The model under review builds one solid part; all positions refer to its coordinate system, in mm. Give positions to 0.01 mm unless a question says otherwise; leave off trailing zeros. Loops run counter-clockwise (first coordinate to the right, second up) from the corner with the lowest first, then second, coordinate; pieces in that order, holes last. Notation, with made-up numbers: (70.5, -19) - (110.5, -19) arc R20 ccw to (110.5, -9) - close; hole circle Ø4 at (44, 28). An arc over 180 degrees is marked (long way). Answer as a JSON object with one key per item and string values.
from build123d import *

# Parameters (mm, degrees)
F1_DEPTH = 1


# Not quite as in the source:
# - ends of sketch curves that miss each other by under 0.0002 mm in the source are joined


with BuildPart() as f1:
    # F0 (on Top) → F1 (new body)
    with BuildSketch(Plane.XY):
        with BuildLine():
            ThreePointArc((5.1893277963, 10.709786768), (5.015248305, 11.2735733528), (4.5536171698, 11.6410725739))
            ThreePointArc((4.5536171698, 11.6410725739), (0, 12.5), (-4.5536171698, 11.6410725739))
            ThreePointArc((-4.5536171698, 11.6410725739), (-5.015248305, 11.2735733528), (-5.1893277963, 10.709786768))
            Line((-5.1893277963, 10.709786768), (-5.1893277963, 10.5791593824))
            ThreePointArc((-5.1893277963, 10.5791593824), (-5.3218672589, 10.0816533863), (-5.6843522286, 9.716025745))
            ThreePointArc((-5.6843522286, 9.716025745), (-7.9596801612, 7.9596801612), (-9.716025745, 5.6843522286))
            ThreePointArc((-9.716025745, 5.6843522286), (-10.0816533863, 5.3218672589), (-10.5791593824, 5.1893277963))
            Line((-10.5791593824, 5.1893277963), (-10.709786768, 5.1893277963))
            ThreePointArc((-10.709786768, 5.1893277963), (-11.2735733528, 5.015248305), (-11.6410725739, 4.5536171698))
            ThreePointArc((-11.6410725739, 4.5536171698), (-12.5, 0), (-11.6410725739, -4.5536171698))
            ThreePointArc((-11.6410725739, -4.5536171698), (-11.2735733528, -5.015248305), (-10.709786768, -5.1893277963))
            Line((-10.709786768, -5.1893277963), (-10.5791593824, -5.1893277963))
            ThreePointArc((-10.5791593824, -5.1893277963), (-10.0816533863, -5.3218672589), (-9.716025745, -5.6843522286))
            ThreePointArc((-9.716025745, -5.6843522286), (-7.9596801612, -7.9596801612), (-5.6843522286, -9.716025745))
            ThreePointArc((-5.6843522286, -9.716025745), (-5.3218672589, -10.0816533863), (-5.1893277963, -10.5791593824))
            Line((-5.1893277963, -10.5791593824), (-5.1893277963, -10.709786768))
            ThreePointArc((-5.1893277963, -10.709786768), (-5.015248305, -11.2735733528), (-4.5536171698, -11.6410725739))
            ThreePointArc((-4.5536171698, -11.6410725739), (0, -12.5), (4.5536171698, -11.6410725739))
            ThreePointArc((4.5536171698, -11.6410725739), (5.015248305, -11.2735733528), (5.1893277963, -10.709786768))
            Line((5.1893277963, -10.709786768), (5.1893277963, -10.5791593824))
            ThreePointArc((5.1893277963, -10.5791593824), (5.3218672589, -10.0816533863), (5.6843522286, -9.716025745))
            ThreePointArc((5.6843522286, -9.716025745), (7.9596801612, -7.9596801612), (9.716025745, -5.6843522286))
            ThreePointArc((9.716025745, -5.6843522286), (10.0816533863, -5.3218672589), (10.5791593824, -5.1893277963))
            Line((10.5791593824, -5.1893277963), (10.709786768, -5.1893277963))
            ThreePointArc((10.709786768, -5.1893277963), (11.2735733528, -5.015248305), (11.6410725739, -4.5536171698))
            ThreePointArc((11.6410725739, -4.5536171698), (12.5, 0), (11.6410725739, 4.5536171698))
            ThreePointArc((11.6410725739, 4.5536171698), (11.2735733528, 5.015248305), (10.709786768, 5.1893277963))
            Line((10.709786768, 5.1893277963), (10.5791593824, 5.1893277963))
            ThreePointArc((10.5791593824, 5.1893277963), (10.0816533863, 5.3218672589), (9.716025745, 5.6843522286))
            ThreePointArc((9.716025745, 5.6843522286), (7.9596801612, 7.9596801612), (5.6843522286, 9.716025745))
            ThreePointArc((5.6843522286, 9.716025745), (5.3218672589, 10.0816533863), (5.1893277963, 10.5791593824))
            Line((5.1893277963, 10.5791593824), (5.1893277963, 10.709786768))
        make_face()
        with BuildLine():
            Line((-1.7389636828, -9.696227699), (-1.7389636828, -7.803772301))
            ThreePointArc((-1.7389636828, -7.803772301), (0, -6.0648086182), (1.7389636828, -7.803772301))
            Line((1.7389636828, -7.803772301), (1.7389636828, -9.696227699))
            ThreePointArc((1.7389636828, -9.696227699), (0, -11.4351913818), (-1.7389636828, -9.696227699))
        make_face(mode=Mode.SUBTRACT)
        with BuildLine():
            Line((-4.0980324058, 1.6278386791), (-4.596886989, 2.1259958547))
            Line((-4.596886989, 2.1259958547), (-7.2887076389, 4.8140532918))
            ThreePointArc((-7.2887076389, 4.8140532918), (-7.2895746597, 7.2895734489), (-4.8140532909, 7.2887076381))
            Line((-4.8140532909, 7.2887076381), (-2.1259958547, 4.596886989))
            Line((-2.1259958547, 4.596886989), (-1.6278386791, 4.0980324058))
            ThreePointArc((-1.6278386791, 4.0980324058), (-1.5783462567, 4.0709813489), (-1.5220880269, 4.0750150967))
            ThreePointArc((-1.5220880269, 4.0750150967), (0.0320676528, 4.349881799), (1.5820019575, 4.052131514))
            Line((1.5820019575, 4.052131514), (2.1259958547, 4.596886989))
            Line((2.1259958547, 4.596886989), (4.8140532909, 7.2887076381))
            ThreePointArc((4.8140532909, 7.2887076381), (7.2895746597, 7.2895734489), (7.2887088489, 4.8140520801))
            Line((7.2887088489, 4.8140520801), (4.596886989, 2.1259958547))
            Line((4.596886989, 2.1259958547), (4.0980324058, 1.6278386791))
            ThreePointArc((4.0980324058, 1.6278386791), (4.0709813489, 1.5783462567), (4.0750150967, 1.5220880269))
            ThreePointArc((4.0750150967, 1.5220880269), (4.35, 0), (4.0750150967, -1.5220880269))
            ThreePointArc((4.0750150967, -1.5220880269), (4.0709813489, -1.5783462567), (4.0980324058, -1.6278386791))
            Line((4.0980324058, -1.6278386791), (4.596886989, -2.1259958547))
            Line((4.596886989, -2.1259958547), (7.2887076389, -4.8140532918))
            ThreePointArc((7.2887076389, -4.8140532918), (7.2904398646, -7.2887076385), (4.8157843062, -7.2904386534))
            Line((4.8157843062, -7.2904386534), (4.8140532909, -7.2887076381))
            Line((4.8140532909, -7.2887076381), (2.1259958547, -4.596886989))
            Line((2.1259958547, -4.596886989), (1.6278386791, -4.0980324058))
            ThreePointArc((1.6278386791, -4.0980324058), (1.5783462567, -4.0709813489), (1.5220880269, -4.0750150967))
            ThreePointArc((1.5220880269, -4.0750150967), (0, -4.35), (-1.5220880269, -4.0750150967))
            ThreePointArc((-1.5220880269, -4.0750150967), (-1.5783462567, -4.0709813489), (-1.6278386791, -4.0980324058))
            Line((-1.6278386791, -4.0980324058), (-2.1259958547, -4.596886989))
            Line((-2.1259958547, -4.596886989), (-4.8140532909, -7.2887076381))
            ThreePointArc((-4.8140532909, -7.2887076381), (-7.2895746597, -7.2895734489), (-7.2887088489, -4.8140520801))
            Line((-7.2887088489, -4.8140520801), (-4.596886989, -2.1259958547))
            Line((-4.596886989, -2.1259958547), (-4.0980324058, -1.6278386791))
            ThreePointArc((-4.0980324058, -1.6278386791), (-4.0709813489, -1.5783462567), (-4.0750150967, -1.5220880269))
            ThreePointArc((-4.0750150967, -1.5220880269), (-4.35, 0), (-4.0750150967, 1.5220880269))
            ThreePointArc((-4.0750150967, 1.5220880269), (-4.0709813489, 1.5783462567), (-4.0980324058, 1.6278386791))
        make_face(mode=Mode.SUBTRACT)
        with BuildLine():
            Line((-7.803772301, -1.7389636828), (-9.696227699, -1.7389636828))
            ThreePointArc((-9.696227699, -1.7389636828), (-11.4351913818, 0), (-9.696227699, 1.7389636828))
            Line((-9.696227699, 1.7389636828), (-7.803772301, 1.7389636828))
            ThreePointArc((-7.803772301, 1.7389636828), (-6.0648086182, 0), (-7.803772301, -1.7389636828))
        make_face(mode=Mode.SUBTRACT)
        with BuildLine():
            Line((9.696227699, -1.7389636828), (7.803772301, -1.7389636828))
            ThreePointArc((7.803772301, -1.7389636828), (6.0648086182, 0), (7.803772301, 1.7389636828))
            Line((7.803772301, 1.7389636828), (9.696227699, 1.7389636828))
            ThreePointArc((9.696227699, 1.7389636828), (11.4351913818, 0), (9.696227699, -1.7389636828))
        make_face(mode=Mode.SUBTRACT)
        with BuildLine():
            Line((1.7389636828, 9.696227699), (1.7389636828, 7.803772301))
            ThreePointArc((1.7389636828, 7.803772301), (0, 6.0648086182), (-1.7389636828, 7.803772301))
            Line((-1.7389636828, 7.803772301), (-1.7389636828, 9.696227699))
            ThreePointArc((-1.7389636828, 9.696227699), (0, 11.4351913818), (1.7389636828, 9.696227699))
        make_face(mode=Mode.SUBTRACT)
    extrude(amount=F1_DEPTH)


solid = f1.part
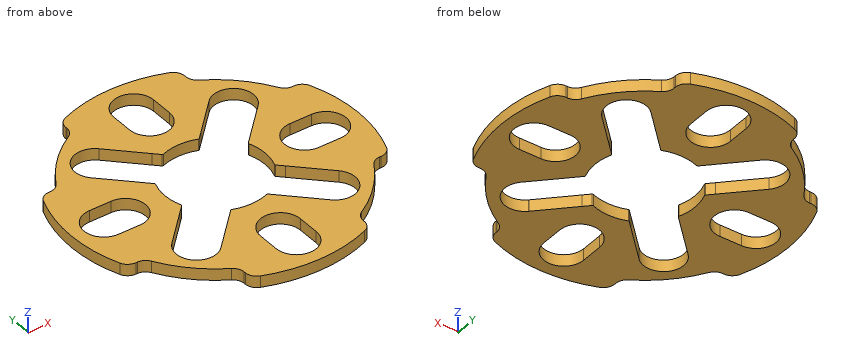
Q1. Consider section C-C, the plane y = 3.5. State the section outline as (x, z) points.
Results:
{"outline": "(-12, 0) - (-5.97, 0) - (-5.97, 1) - (-12, 1) - close; (5.97, 0) - (12, 0) - (12, 1) - (5.97, 1) - close"}
Q2. To check wall thickness, follow probe 1 along Y at (x, z) = (0.5, 0.15); probe 2 along Y at (x, z) = (4.75, 0.45); probe 3 along Y at (x, z) = (-6, 0.35). State the ranges of each line that lie inside material, in increasing order. Write a range as [from, to].
Results:
{"probe 1": "y = [-12.49, -11.36], [-6.14, -4.32], [4.32, 6.14], [11.36, 12.49]", "probe 2": "y = [-11.54, -7.22], [-2.28, 2.28], [7.22, 11.54]", "probe 3": "y = [-9.52, -7.8], [-3.53, 3.53], [7.8, 9.52]"}
Q3. Consider section D-D, the plane z = 0.7. State how many separate pieces and enclosed holes the cut face has, plus the area to 3 significant figures.
Results:
{"separate pieces": "1", "enclosed holes": "5", "area": "248 mm^2"}
Q4. Consider section A-A, the plane y = 0. State the section outline as (x, z) points.
Results:
{"outline": "(-12.5, 0) - (-11.44, 0) - (-11.44, 1) - (-12.5, 1) - close; (-6.06, 0) - (-4.35, 0) - (-4.35, 1) - (-6.06, 1) - close; (4.35, 0) - (6.06, 0) - (6.06, 1) - (4.35, 1) - close; (11.44, 0) - (12.5, 0) - (12.5, 1) - (11.44, 1) - close"}
